Geometry check sheet. Reference: the model listing, model coordinates, mm. Coordinates: 2 decimals unless noted, no trailing zeros. Write each loop counter-clockwise with the first axis right and the second up, starting at its lowest first coordinate (ties: lowest second). Pieces come first, ordered by that corner, then holes. Notation, with made-up numbers: M 22.25,-11 L 49.25,-11 A23 cw 49.25,4 Z; hole C 69,-1.5 d11. An arc over 180 degrees is marked long. Put each result on its own line as item: value. Start each with the question number.
1) Cross-section at D-D on z = -17. Record the cut outline in (x, y), plus the area to 3 significant figures.
2) Gauge pin test, flat ends, axial feed: pin 1 (0.6 mm diameter, centred on x = 0.5, y = -0.5, fed in from -Z); pin 2 (1 mm diameter, centred on x = 0.5, y = -18, fed in from -Z). Record the tip position at first contact, or that the pin passes through.
3) Cross-section at A-A on x = 0. Record the cut outline in (y, z).
4) Cross-section at C-C on y = -28. Record the cut outline in (x, z), plus the area to 3 significant figures.
5) Scan lines: line 1 along Y through (x, z) = (0.05, 25.5); line 2 along Y through (x, z) = (0.75, 26); line 3 along Z through (x, y) = (0.6, -23). Record each from-to range of solid material in increasing order.
6) Cross-section at B-B on z = 7.5. Record the cut outline in (x, y), plus the area to 3 significant figures.
from build123d import *

# Parameters (mm, degrees)
BARRER1_PROFILE_R = 1


with BuildPart() as part:
    # Barrer1: sweep along a path in Croquis1
    with BuildLine(Plane(origin=(0, 0, 0), x_dir=(0, 0, -1), z_dir=(1, 0, 0))) as barrer1_path:
        Line((0, 0), (-32.66, 0))
        ThreePointArc((-32.66, 0), (-34.074213562, -0.585786438), (-34.66, -2))
        Line((-34.66, -2), (-34.66, -102.36))
        ThreePointArc((-34.66, -102.36), (-34.074213562, -103.774213562), (-32.66, -104.36))
        Line((-32.66, -104.36), (19.69, -104.36))
        ThreePointArc((19.69, -104.36), (21.104213562, -104.945786438), (21.69, -106.36))
        Line((21.69, -106.36), (21.69, -121.36))
    # Barrer1 profile (on start of the path) → Barrer1 (sweep)
    with BuildSketch(Plane(origin=(0, 0, 0), x_dir=(0, 1, 0), z_dir=(0, 0, 1))):
        Circle(BARRER1_PROFILE_R)
    sweep(path=barrer1_path.line)


solid = part.part
Answer key:
1. outline: C 0,-104.36 d2
1. area: 3.14 mm²
2. pin 1: stops at z = 0
2. pin 2: stops at z = 33.66
3. outline: M -121.36,-22.69 L -106.36,-22.69 A3 ccw -103.36,-19.69 L -103.36,32.66 A1 cw -102.36,33.66 L -2,33.66 A1 cw -1,32.66 L -1,0 L 1,0 L 1,32.66 A3 ccw -2,35.66 L -102.36,35.66 A3 ccw -105.36,32.66 L -105.36,-19.69 A1 cw -106.36,-20.69 L -121.36,-20.69 Z
4. outline: C 0,34.66 d2
4. area: 3.14 mm²
5. line 1: y = -105.36 to -103.36, -1 to 1
5. line 2: y = -105.02 to -103.7, -0.66 to 0.66
5. line 3: z = 33.86 to 35.46
6. outline: C 0,-104.36 d2; C 0,0 d2
6. area: 6.28 mm²
